from build123d import *

# Parameters (mm, degrees)
SKETCH1_W               = 11
SKETCH1_H               = 10
BOSS_EXTRUDE1_DEPTH     = 1.5
SKETCH3_W               = 3
SKETCH3_H               = 4
BOSS_EXTRUDE2_DEPTH     = 1.5
CUT_EXTRUDE1_DEPTH      = 10.974968672
CUT_EXTRUDE1_DEPTH_BACK = 10.974968672
SKETCH4_R               = 2.1


with BuildPart() as part:
    # Sketch1 → Boss-Extrude1 (new, symmetric)
    with BuildSketch(Plane.XY):
        Rectangle(SKETCH1_W, SKETCH1_H)
    extrude(amount=BOSS_EXTRUDE1_DEPTH, both=True)

    # Sketch3 → Boss-Extrude2 (add, symmetric)
    with BuildSketch(Plane.XY):
        with Locations((-7, 0)):
            Rectangle(SKETCH3_W, SKETCH3_H)
        with Locations((7, 0)):
            Rectangle(SKETCH3_W, SKETCH3_H)
    extrude(amount=BOSS_EXTRUDE2_DEPTH, both=True)

    # Sketch4 → Cut-Extrude1 (cut, two sides: drawn at the far end of the back side and taken through both)
    with BuildSketch(Plane.XY.offset(-CUT_EXTRUDE1_DEPTH_BACK)):
        Circle(SKETCH4_R)
    extrude(amount=CUT_EXTRUDE1_DEPTH + CUT_EXTRUDE1_DEPTH_BACK, mode=Mode.SUBTRACT)


solid = part.part
Source: CAD feature listing. Evaluate the final solid. Frame: model axes, mm. A direction names the side the tool comes from. Give positions to 0.01 mm unless a question says otherwise; leave off trailing zeros. Write each loop counter-clockwise with the first axis right and the second up, starting at its lowest first coordinate (ties: lowest second). Pieces come first, ordered by that corner, then holes. Notation, with made-up numbers: M 12.25,26.25 L 18.25,26.25 A22 cw 18.25,60.25 Z; hole C 46.25,72 d5. An arc over 180 degrees is marked long. Return JSON: item names as keys, results as strings. Group by question number.
1) First-contact query: pin 1 Ø0.9 at (x, z) = (-7.5, 0) entering from -Y; pin 2 Ø1 at (y, z) = (4, 0) entering from +X; pin 3 Ø1.5 at (x, z) = (7, 0.5) entering from +Y; pin 4 Ø2.5 at (x, y) = (0, 0) entering from +Z. Flat tips, straight axial feed; report the tip coordinate or a pass-through.
2) Set-up query: faces 4 (the face through (-5.5, -4, 0)), 5 (the face through (7, -2, 0)), 6 (the face through (-7, 2, 0)). Return all of +Z, -Z, +X, -X, +Y, -Y with unobstructed straight access to the full face (end or side cutting, diameter ignored); none if empty.
3) Cut plane B-B, the plane x = -0.5. Output: boundary loops of the cut face in (y, z).
4) Cut plane A-A, the plane y = 1. Output: boundary loops of the cut face in (x, z), then the cut area to 3 significant figures.
5) Cut plane D-D, the plane y = -4. Output: boundary loops of the cut face in (x, z).
6) Ray query, L1, parallel to Y at x = 0, z = 0.1; L2, parallel to X at y = 0, z = -0.15; L3, parallel to Y at x = -7.75, z = 0. Return the intervals inside material, ascending.
7) Cut plane C-C, the plane z = 0.7. Output: boundary loops of the cut face in (x, y).
8) Draft query along X for faces 1 (the face through (2.003, 0.631, -0.021)), 2 (the face through (-2, 1.2, -1.5)), 3 (the face through (5.5, 3, 0)). Return one class per face: released by +X, released by -X, zero draft, split by the parting line, or undercut.
Data:
{
 "1": {"pin 1": "stops at y = -2", "pin 2": "stops at x = 5.5", "pin 3": "stops at y = 2", "pin 4": "passes through"},
 "2": {"face 4": "+Z, -Z, -X, -Y", "face 5": "+Z, -Z, +X, -Y", "face 6": "+Z, -Z, -X, +Y"},
 "3": {"outline": "M -5,-1.5 L -2.04,-1.5 L -2.04,1.5 L -5,1.5 Z; M 2.04,-1.5 L 5,-1.5 L 5,1.5 L 2.04,1.5 Z"},
 "4": {"outline": "M -8.5,-1.5 L -1.85,-1.5 L -1.85,1.5 L -8.5,1.5 Z; M 1.85,-1.5 L 8.5,-1.5 L 8.5,1.5 L 1.85,1.5 Z", "area": "39.9 mm²"},
 "5": {"outline": "M -5.5,-1.5 L 5.5,-1.5 L 5.5,1.5 L -5.5,1.5 Z"},
 "6": {"L1": "y = -5 to -2.1, 2.1 to 5", "L2": "x = -8.5 to -2.1, 2.1 to 8.5", "L3": "y = -2 to 2"},
 "7": {"outline": "M -8.5,-2 L -5.5,-2 L -5.5,-5 L 5.5,-5 L 5.5,-2 L 8.5,-2 L 8.5,2 L 5.5,2 L 5.5,5 L -5.5,5 L -5.5,2 L -8.5,2 Z; hole C 0,0 d4.2"},
 "8": {"face 1": "undercut", "face 2": "zero draft", "face 3": "released by +X"}
}
